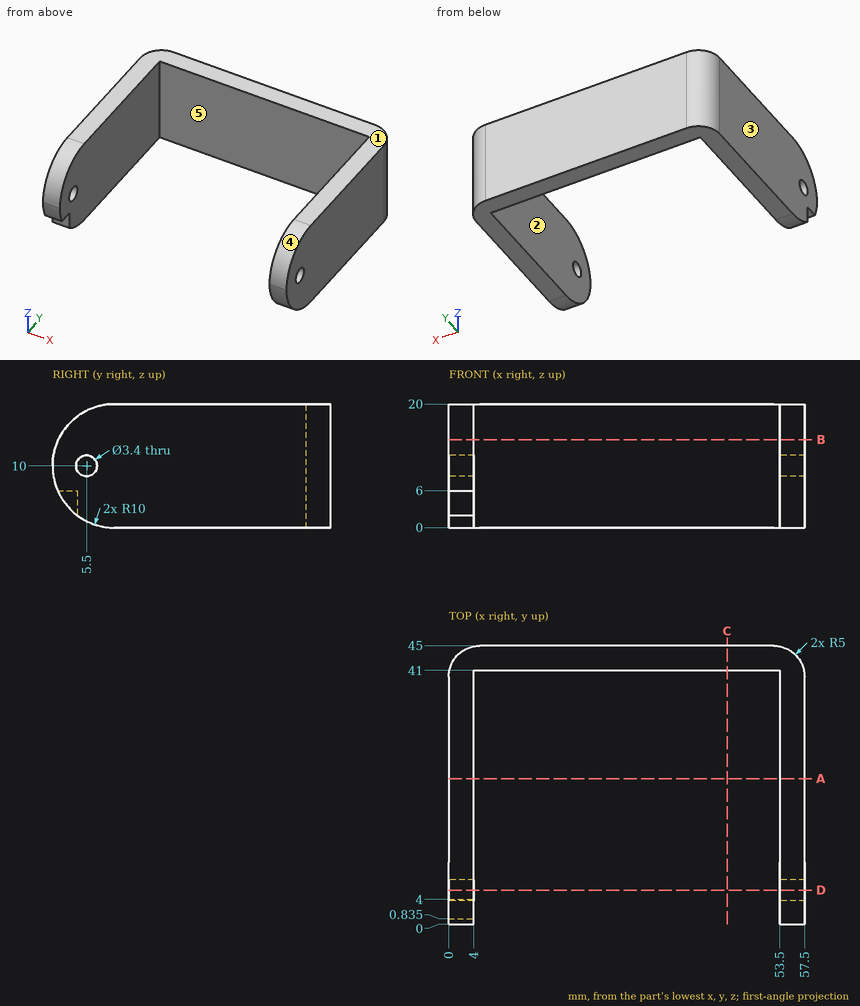
Can you work these out from the drawing? Everything is in mm from the part's minimum corner. A direction names the side the tool comes from. Give positions to 0.01 mm unless a question says otherwise; leave off trailing zeros. Order: outer loops, then holes, each group sorted by start corner. A loop starts at its lowest first (then second) coordinate and runs counter-clockwise, first axis right, second up. Notation, with made-up numbers: M 79.5,16 L 113.5,16 A8 cw 113.5,24 Z; hole C -9.5,77.25 d5. An arc over 180 degrees is marked long. Use a Markdown table: item, result. Add a question column.
Item 1: Suppose I cut it at A-A (y = 23.5). List the corners of the cut face in (x, z) for me, then the cut area to 3 significant figures.
Item 2: Suppose I cut it at C-C (x = 45). List the corners of the cut face in (y, z) for me, then the cut area to 3 significant figures.
Item 3: Suppose I cut it at D-D (y = 5.5). List the corners of the cut face in (x, z) for me, then the cut area to 3 significant figures.
Item 4: Will these pins go through, and if not, where does the flat tip stop? pin 1 (3 mm diameter, centred on y = 5.5, z = 10, fed in from +X) (1 decimal); pin 2 (12 mm diameter, centred on x = 28, z = 15.5, fed in from -Y); pin 3 (3.5 mm diameter, centred on x = 2.5, y = 3, fed in from -Z); pin 4 (1.2 mm diameter, centred on x = 2.5, z = 5, fed in from -Y).
Item 5: Suppose I cut it at B-B (z = 14.25). List the corners of the cut face in (x, y) for me.
Item 6: For the marked faces 4 and 5, which set-ups out of +Z, -Z, +X, -X, +Y, -Y let a thin tool reach every point of the face, with its end or its side?
Item 7: If I drill on L1, parallel to X at y = 24, z = 6.75; L2, parallel to Y at x = 50, z = 11; L3, parallel to Y at x = 54.95, z = 10, over which ranges is the centre line in solid material (lowest first)? Write a range as [from, to].
Item 8: We'd pull the mould along X, two halves only. Please class the marked faces 1, 2 and 3: +X half, -X half, draft (parallel to the pull), parting line (faces both ways), or undercut.
Answer sheet:
| question | item | result |
|---|---|---|
| 1 | outline | M 0,0 L 4,0 L 4,20 L 0,20 Z; M 53.5,0 L 57.5,0 L 57.5,20 L 53.5,20 Z |
| 1 | area | 160 mm² |
| 2 | outline | M 41,0 L 45,0 L 45,20 L 41,20 Z |
| 2 | area | 80.0 mm² |
| 3 | outline | M 0,1.07 L 4,1.07 L 4,8.3 L 0,8.3 Z; M 0,11.7 L 4,11.7 L 4,18.93 L 0,18.93 Z; M 53.5,1.07 L 57.5,1.07 L 57.5,8.3 L 53.5,8.3 Z; M 53.5,11.7 L 57.5,11.7 L 57.5,18.93 L 53.5,18.93 Z |
| 3 | area | 116 mm² |
| 4 | pin 1 | passes through |
| 4 | pin 2 | stops at y = 41 |
| 4 | pin 3 | stops at z = 1.49 |
| 4 | pin 4 | stops at y = 4 |
| 5 | outline | M 0,0.95 L 4,0.95 L 4,41 L 53.5,41 L 53.5,0.95 L 57.5,0.95 L 57.5,40 A5 ccw 52.5,45 L 5,45 A5 ccw 0,40 Z |
| 6 | face 4 | +Z, +X, -X, -Y |
| 6 | face 5 | +Z, -Z, -Y |
| 7 | L1 | x = [0, 4], [53.5, 57.5] |
| 7 | L2 | y = [41, 45] |
| 7 | L3 | y = [0, 3.8], [7.2, 44.36] |
| 8 | face 1 | draft |
| 8 | face 2 | undercut |
| 8 | face 3 | -X half |
